For this review, take the finished solid that the model builds, in its own axes (mm). A direction names the side the tool comes from. Coordinates: 2 decimals unless noted, no trailing zeros. Write each loop counter-clockwise with the first axis right and the second up, starting at its lowest first coordinate (ties: lowest second). Pieces come first, ordered by that corner, then holes.
1) Mouldability with a two-part tool opening along Y and no side actions: class faces 1 (the face through (13.9, 15.57, 1.48)), 2 (the face through (18.4, 0.3, 0)), 3 (the face through (-20, -19, 2)) as pulls with the +Y half, pulls with the -Y half, needs draft (parallel to the pull), parting line crosses it, or undercut.
2) We need section D-D on y = 15.5. Write out the cut boundary in (x, z).
3) Insertion check: P1, Ø12.5, axis at x = 0, y = 7, coming from the -Z side; P2, Ø2.5, axis at x = -15.5, y = -15.5, coming from the +Z side; P3, Ø4, axis at x = -2.5, z = -5.5, coming from the -Y side; P4, Ø2, axis at x = -12.5, z = -3.5, coming from the +Y side. Each pin has a flat end and moves straight along its axis. Give the tip position at first contact, or say it passes through.
4) We need section A-A on z = 0.75. Write out the cut boundary in (x, y), then the cut area to 3 significant figures.
5) To check wall thickness, follow line 1 along Y through (x, z) = (15.5, 2.05); line 2 along Y through (x, z) = (0, -3); line 3 along Z through (x, y) = (-16.5, 13). State the ranges of each line that lie inside material, in increasing order.
6) We need section B-B on x = 0. Write out the cut boundary in (y, z).
7) For faces 4 (the face through (19, 20, 2)), 5 (the face through (3.47, -15.62, -3.45)), list the 3-axis set-ups (+Z, -Z, +X, -X, +Y, -Y) from which the entire face can be reached by the end or side of a thin tool; tool diameter is ignored.
from build123d import *

# Parameters (mm, degrees)
SKETCH_1_W      = 42
SKETCH_1_H      = 42
SKETCH_1_R      = 1.6
SKETCH_1_R_2    = 11
EXTRUDE_1_DEPTH = 3
FILLET_1_R      = 5
SKETCH_2_R      = 18
SKETCH_2_R_2    = 16
EXTRUDE_2_DEPTH = 7


with BuildPart() as part:
    # 草图1 → 凸台-拉伸1 (new body)
    with BuildSketch(Plane.XY):
        Rectangle(SKETCH_1_W, SKETCH_1_H)
        with Locations((-15.5, 15.5)):
            Circle(SKETCH_1_R, mode=Mode.SUBTRACT)
        with Locations((15.5, 15.5)):
            Circle(SKETCH_1_R, mode=Mode.SUBTRACT)
        with Locations((15.5, -15.5)):
            Circle(SKETCH_1_R, mode=Mode.SUBTRACT)
        with Locations((-15.5, -15.5)):
            Circle(SKETCH_1_R, mode=Mode.SUBTRACT)
        Circle(SKETCH_1_R_2, mode=Mode.SUBTRACT)
    extrude(amount=EXTRUDE_1_DEPTH)

    # 圆角1
    fillet_1_edges = [part.edges().sort_by_distance(p)[0] for p in [
        (-21, -21, 1.5),
        (-21, 21, 1.5),
        (21, 21, 1.5),
        (21, -21, 1.5),
    ]]
    fillet(fillet_1_edges, radius=FILLET_1_R)

    # 草图2 → 凸台-拉伸2 (add)
    with BuildSketch(Plane(origin=(0, 0, 0), x_dir=(-1, 0, 0), z_dir=(0, 0, -1))):
        with Locations(Location((0, 0, 0), (0, 0, 180))):
            Circle(SKETCH_2_R)
        Circle(SKETCH_2_R_2, mode=Mode.SUBTRACT)
    extrude(amount=EXTRUDE_2_DEPTH)


solid = part.part
Result:
1. face 1: undercut
1. face 2: needs draft
1. face 3: pulls with the -Y half
2. outline: (-21, 0) - (-17.1, 0) - (-17.1, 3) - (-21, 3) - close; (-13.9, 0) - (-9.15, 0) - (-9.15, -7) - (-3.97, -7) - (-3.97, 0) - (3.97, 0) - (3.97, -7) - (9.15, -7) - (9.15, 0) - (13.9, 0) - (13.9, 3) - (-13.9, 3) - close; (17.1, 0) - (21, 0) - (21, 3) - (17.1, 3) - close
3. P1: stops at z = 0
3. P2: passes through
3. P3: stops at y = -17.99
3. P4: stops at y = 13.85
4. outline: (-21, -16) arc R5 ccw to (-16, -21) - (16, -21) arc R5 ccw to (21, -16) - (21, 16) arc R5 ccw to (16, 21) - (-16, 21) arc R5 ccw to (-21, 16) - close; hole circle Ø3.2 at (-15.5, -15.5); hole circle Ø3.2 at (-15.5, 15.5); hole circle Ø22 at (0, 0); hole circle Ø3.2 at (15.5, -15.5); hole circle Ø3.2 at (15.5, 15.5)
4. area: 1,330 mm2
5. line 1: y = -21 to -17.1, -13.9 to 13.9, 17.1 to 21
5. line 2: y = -18 to -16, 16 to 18
5. line 3: z = 0 to 3
6. outline: (-21, 0) - (-18, 0) - (-18, -7) - (-16, -7) - (-16, 0) - (-11, 0) - (-11, 3) - (-21, 3) - close; (11, 0) - (16, 0) - (16, -7) - (18, -7) - (18, 0) - (21, 0) - (21, 3) - (11, 3) - close
7. face 4: +Z, -Z, +X, +Y
7. face 5: -Z
